```python
from build123d import *

# Parameters (mm, degrees)
ESQUISSE2_R             = 2.5
BOSS_EXTRU_1_DEPTH      = 10
BOSS_EXTRU_1_DEPTH_BACK = 10
ESQUISSE3_R             = 5
ESQUISSE3_R_2           = 2.5
ESQUISSE5_R             = 2.5
ENL_V_MAT_EXTRU_1_DEPTH = 143.711247056


with BuildPart() as part:
    # Balayage1: sweep along a path in Esquisse1
    with BuildLine(Plane.XY) as balayage1_path:
        Line((0, 127), (0, 137))
        Line((0, 137), (15, 137))
        ThreePointArc((15, 137), (18.535533906, 135.535533906), (20, 132))
        Line((20, 132), (20, 5))
        ThreePointArc((20, 5), (18.535533906, 1.464466094), (15, 0))
        Line((15, 0), (0, 0))
        Line((0, 0), (0, 10))
    # Esquisse2 → Balayage1 (sweep)
    with BuildSketch(Plane(origin=(0, 127, 0), x_dir=(1, 0, 0), z_dir=(0, 1, 0))):
        Circle(ESQUISSE2_R)
    sweep(path=balayage1_path.line, transition=Transition.RIGHT)

    # Esquisse3 → Boss.-Extru.1 (add, two sides: drawn at the far end of the back side and taken through both)
    # profile 1 of 2: a face of its own
    with BuildSketch(Plane.XY.offset(-BOSS_EXTRU_1_DEPTH_BACK)):
        with Locations((0, 127)):
            Circle(ESQUISSE3_R)
        with Locations((0, 127)):
            Circle(ESQUISSE3_R_2, mode=Mode.SUBTRACT)
    # profile 2 of 2: a face of its own
    with BuildSketch(Plane.XY.offset(-BOSS_EXTRU_1_DEPTH_BACK)):
        with Locations((0, 10)):
            Circle(ESQUISSE3_R)
        with Locations((0, 10)):
            Circle(ESQUISSE3_R_2, mode=Mode.SUBTRACT)
    extrude(amount=BOSS_EXTRU_1_DEPTH + BOSS_EXTRU_1_DEPTH_BACK)

    # Esquisse5 → Enlèv. mat.-Extru.1 (cut, through all)
    with BuildSketch(Plane.XY.offset(10)):
        with Locations((0, 127)):
            Circle(ESQUISSE5_R)
        with Locations((0, 10)):
            Circle(ESQUISSE5_R)
    extrude(amount=-ENL_V_MAT_EXTRU_1_DEPTH, mode=Mode.SUBTRACT)


solid = part.part
```
Could you check a few things on this model? Use its own coordinates, in mm. A direction names the side the tool comes from. Coordinates: 2 decimals unless noted, no trailing zeros. Order: outer loops, then holes, each group sorted by start corner. A loop starts at its lowest first (then second) coordinate and runs counter-clockwise, first axis right, second up. Notation, with made-up numbers: M -0.5,2 L 55.5,2 A20 cw 55.5,15 Z; hole C -21.75,-5 d6. An arc over 180 degrees is marked long. Use one line per item in the form item = value. Start each with the question number.
1. Suppose I cut it at D-D on z = -8. Write out the boundary of the cut face in (x, y).
2. Please list where these lines run through material, in increasing order: line 1 (Y direction, x = 0, z = 3.5); line 2 (Y direction, x = -0.5, z = -5.75); line 3 (X direction, y = 123, z = 2).
3. On a 3-axis mill with a long thin cutter (end or side, diameter ignored), from which of +Z, -Z, +X, -X, +Y, -Y can I reach the whole of each face in a straight line? I mean faces 3 (the cylindrical face through (-2.5, 134.6, -0.1)), 4 (the cylindrical face through (1.34, 129.11, -0.14)). Say none if no direction works.
4. We'd pull the mould along X, two halves only. Please class faces 1 (the cylindrical face through (-0.54, 7.56, -0.14)), 2 (the flat face through (2, 125, 10)): +X half, -X half, draft (parallel to the pull), parting line (faces both ways), or undercut.
5. Suppose I cut it at C-C on z = 0. Write out the boundary of the cut face in (x, y), then the cut area to 3 significant figures.
6. Suppose I cut it at A-A on x = 0. Write out the boundary of the cut face in (y, z).
7. For pin 1 (10 mm diameter, centred on x = 15, y = 24.5, fed in from -Z); pin 2 (10 mm diameter, centred on y = 68, z = 4.5, fed in from -X); pin 3 (1.5 mm diameter, centred on y = 78, z = -3, fed in from -X); pin 4 (4 mm diameter, centred on y = 18.5, z = -5.5, fed in from +X), each with a flat end and sliding along its axis, tell me the tip position at first contact or that it passes through.
8. Suppose I cut it at B-B on y = 10. Write out the boundary of the cut face in (x, z).
Geometry says:
q1.outline = C 0,10 d10; C 0,127 d10; hole C 0,10 d5; hole C 0,127 d5
q2.line_1 = 5 to 7.5, 12.5 to 15, 122 to 124.5, 129.5 to 132
q2.line_2 = 5.03 to 7.55, 12.45 to 14.97, 122.03 to 124.55, 129.45 to 131.97
q2.line_3 = -3 to 3, 18.5 to 21.5
q3.face_3 = none
q3.face_4 = +Z, -Z
q4.face_1 = undercut
q4.face_2 = draft
q5.outline = M -2.5,-2.5 L 15,-2.5 A7.5 ccw 22.5,5 L 22.5,132 A7.5 ccw 15,139.5 L -2.5,139.5 L -2.5,131.33 A5 ccw long 2.5,131.33 L 2.5,134.5 L 15,134.5 A2.5 cw 17.5,132 L 17.5,5 A2.5 cw 15,2.5 L 2.5,2.5 L 2.5,5.67 A5 ccw long -2.5,5.67 Z; hole C 0,10 d5; hole C 0,127 d5
q5.area = 1,030 mm^2
q6.outline = M 0,-2.5 L 5,-2.5 L 5,-10 L 7.5,-10 L 7.5,10 L 5,10 L 5,2.5 L 0,2.5 A2.5 ccw Z; M 12.5,-10 L 15,-10 L 15,10 L 12.5,10 Z; M 122,-10 L 124.5,-10 L 124.5,10 L 122,10 Z; M 129.5,-10 L 132,-10 L 132,-2.5 L 137,-2.5 A2.5 ccw 137,2.5 L 132,2.5 L 132,10 L 129.5,10 Z
q7.pin_1 = -2.5
q7.pin_2 = 17.5
q7.pin_3 = 18.91
q7.pin_4 = through
q8.outline = M -5,-10 L -2.5,-10 L -2.5,10 L -5,10 Z; M 2.5,-10 L 5,-10 L 5,10 L 2.5,10 Z; C 20,0 d5
